Autodesk Inventor part; units mm, degrees
ref_plane "工作平面1" through (0, 165, 525) normal (0, 1, 0) x (1, 0, 0)
ref_plane "工作平面2" through (0, -340, 225) normal (0, 0, 1) x (1, 0, 0)
ref_plane "工作平面3" through (125, 0, 0) normal (1, 0, 0) x (0, 0, -1)
sketch "草图1" plane through (0, 0, 0) normal (1, 0, 0) x (0, 1, 0)
  line L0 (340, -525) -> (-340, -525)
  line L1 (-340, -525) -> (-340, 525)
  line L2 (-340, 525) -> (340, 525)
  line L3 (340, 525) -> (340, -525)
  line L4 (340, -525) -> (-340, 525) construction
  line L5 (-340, -525) -> (340, 525) construction
  point P0 (0, 0)
  dimension "d0" = 680
  dimension "d1" = 1050
extrude "拉伸1" add sketch "草图1" along normal blind 190
fillet "圆角1" [suppressed]
sketch "草图2" plane through (190, 0, 0) normal (1, 0, 0) x (0, 0, -1)
  line L0 (475, -290) -> (-475, -290)
  line L1 (475, 290) -> (475, -290)
  line L2 (-475, 290) -> (475, 290)
  line L3 (-475, -290) -> (-475, 290)
  line L4 (-475, 290) -> (475, 290)
  line L5 (475, 290) -> (475, 190)
  line L6 (475, 190) -> (-475, 190)
  line L7 (-475, 190) -> (-475, 290)
  point P0 (0, 0)
  dimension "d5" = 100
extrude "拉伸2" [suppressed]
sketch "草图3" plane through (190, 0, 0) normal (1, 0, 0) x (0, 0, -1)
  line L0 (-475, -290) -> (-475, 290)
  line L1 (475, -290) -> (-475, -290)
  line L2 (475, 290) -> (475, -290)
  line L3 (-525, -340) -> (525, -340)
  line L4 (-525, 340) -> (-525, -340)
  line L5 (525, -340) -> (525, 340)
  line L6 (-475, -241.0052) -> (375, -241.0052)
  line L7 (375, -241.0052) -> (375, -341.0052)
  line L8 (375, -341.0052) -> (-475, -341.0052)
  line L9 (-475, -341.0052) -> (-475, -241.0052)
  point P0 (0, 0)
  point P1 (425, -191.0052)
  point P2 (425, -240)
  dimension "d8" = 850
  dimension "d9" = 100
extrude "拉伸3" [suppressed]
sketch "草图4" plane through (190, -191.0052, -425) normal (0, -1, 0) x (1, 0, 0)
  line L0 (-27.3454, 1.363) -> (-107.3454, 1.363)
  line L1 (-107.3454, 1.363) -> (-107.3454, 851.363)
  line L2 (-107.3454, 851.363) -> (-27.3454, 851.363)
  line L3 (-27.3454, 851.363) -> (-27.3454, 1.363)
  point P0 (-190, 425)
  dimension "d12" = 80
  dimension "d13" = 850
extrude "拉伸4" [suppressed]
sketch "草图5" plane through (190, 0, 0) normal (1, 0, 0) x (0, 0, -1)
  line L0 (475, -290) -> (-475, -290)
  line L1 (475, 290) -> (475, -290)
  line L2 (-475, 290) -> (475, 290)
  line L3 (-475, -290) -> (-475, 290)
  line L4 (-400, -285) -> (400, -285)
  line L5 (400, -285) -> (400, -325)
  line L6 (400, -325) -> (-400, -325)
  line L7 (-400, -325) -> (-400, -285)
  line L8 (-525, -340) -> (525, -340)
  point P0 (0, 0)
  point P1 (-400, -305)
  point P2 (-400, -290)
  point P3 (400, -290)
  dimension "d16" = 800
  dimension "d17" = 40
  dimension "d19" = 75
  dimension "d34" = 55
extrude "拉伸5" cut sketch "草图5" against normal blind 105 contours L5 L6 L7 L0 | L0 L7 L4 L5
ref_plane "工作平面1" through (0, 165, 525) normal (0, 1, 0) x (1, 0, 0)
sketch "草图6" plane through (0, 165, 525) normal (0, 1, 0) x (1, 0, 0)
  line L0 (190, 50) -> (190, 1000)
  arc A0 (190, 1000) -> (140, 1050) centre (140, 1000) ccw
  line L1 (140, 1050) -> (140, 0)
  arc A1 (140, 0) -> (190, 50) centre (140, 50) ccw
  line L2 (0, 1050) -> (190, 1050)
  line L3 (0, 1050) -> (0, 0)
  line L4 (0, 0) -> (190, 0)
  line L5 (145, 150) -> (45, 150)
  line L6 (45, 150) -> (45, 900)
  line L7 (45, 900) -> (145, 900)
  line L8 (145, 900) -> (145, 150)
  line L9 (190, 1050) -> (190, 0)
  point P0 (0, 525)
  dimension "d23" = 100
  dimension "d24" = 750
  dimension "d25" = 150
  dimension "d26" = 45
extrude "拉伸6" cut sketch "草图6" against normal blind 450 contours L5 L6 L7 L1 | L1 L7 L8 L5
fillet "圆角3" [suppressed]
ref_plane "工作平面2" through (0, -340, 225) normal (0, 0, 1) x (1, 0, 0)
sketch "草图7" plane through (0, -340, 225) normal (0, 0, 1) x (1, 0, 0)
  point P0 (0, 340)
sketch "草图8" plane through (0, -340, 225) normal (0, 0, 1) x (1, 0, 0)
  line L0 (-8.4267, 713.5838) -> (252.801, 713.5838)
  line L1 (252.801, 713.5838) -> (252.801, -46.692)
  line L2 (252.801, -46.692) -> (-8.4267, -46.692)
  line L3 (-8.4267, -46.692) -> (-8.4267, 713.5838)
  point P0 (0, 340)
extrude "拉伸7" [suppressed]
sketch "草图9" plane through (190, -285, -400) normal (0, -1, 0) x (1, 0, 0)
  line L0 (0, 800) -> (-105, 800)
  line L1 (0, 0) -> (-105, 0)
  line L2 (-105, 0) -> (-105, 800)
  arc A0 (0, 875) -> (-50, 925) centre (-50, 875) ccw
  line L3 (0, 875) -> (-190, 875)
  line L4 (-190, -125) -> (-190, 925)
  arc A1 (-50, -125) -> (0, -75) centre (-50, -75) ccw
  line L5 (0, -75) -> (-190, -75)
  line L6 (-95, 875) -> (-95, -75)
  line L7 (-25, 800) -> (-65, 800)
  line L8 (-65, 800) -> (-65, 0)
  line L9 (-65, 0) -> (-25, 0)
  line L10 (-25, 0) -> (-25, 800)
  line L11 (-185, 800) -> (-145, 800)
  line L12 (-145, 800) -> (-145, 0)
  line L13 (-145, 0) -> (-185, 0)
  line L14 (-185, 0) -> (-185, 800)
  point P0 (-190, 400)
  point P1 (-14.2929, 800)
  point P2 (-14.2929, 0)
  point P3 (-25, 0)
  point P4 (-65, 800)
  dimension "d35" = 40
  dimension "d36" = 30
extrude "拉伸8" [suppressed]
ref_plane "工作平面3" through (125, 0, 0) normal (1, 0, 0) x (0, 0, -1)
sketch "草图10" plane through (125, 0, 0) normal (1, 0, 0) x (0, 0, -1)
  line L0 (400, -280) -> (-400, -280)
  line L1 (-400, -280) -> (-400, 220)
  line L2 (-400, 220) -> (400, 220)
  line L3 (400, -280) -> (400, 220)
  line L4 (-400, 220) -> (400, 220)
  line L5 (400, 220) -> (400, 160)
  line L6 (400, 160) -> (-400, 160)
  line L7 (-400, 160) -> (-400, 220)
  point P0 (0, 0)
  point P1 (-400, 160)
  point P2 (400, 160)
  dimension "d40" = 800
  dimension "d41" = 60
extrude "拉伸9" [suppressed]
fillet "圆角4" [suppressed]
ref_plane "工作平面4" through (190, -290, -400) normal (0, -1, 0) x (1, 0, 0)
ref_plane "工作平面5" through (95, 0, 0) normal (1, 0, 0) x (0, 0, -1)
ref_plane "工作平面6" through (190, -290, 350) normal (0, 0, -1) x (-1, 0, 0)
sketch "草图11" plane through (0, -340, -525) normal (0, 0, -1) x (-1, 0, 0)
  point P0 (0, 340)
ref_plane "工作平面7" through (0, -340, 225) normal (0, 0, 1) x (1, 0, 0)
sketch "草图12" plane through (0, -340, 225) normal (0, 0, 1) x (1, 0, 0)
  line L0 (145, 505) -> (45, 505)
  line L1 (145, 55) -> (85, 55)
  line L2 (145, 505) -> (145, 55)
  line L3 (145, 505) -> (45, 505)
  line L4 (45, 505) -> (45, 55)
  line L5 (45, 55) -> (85, 55)
  line L6 (190, 55) -> (190, 15)
  line L7 (190, 55) -> (85, 55)
  line L8 (85, 55) -> (85, 15)
  line L9 (190, 15) -> (85, 15)
  line L10 (0, 0) -> (190, 0)
  line L11 (0, 0) -> (0, 680)
  line L12 (0, 680) -> (190, 680)
  line L13 (190, 0) -> (190, 680)
  point P0 (0, 340)
sketch "草图13" plane through (0, -340, -525) normal (0, 0, -1) x (-1, 0, 0)
  line L0 (-45, 505) -> (-45, 55)
  line L1 (-45, 55) -> (-85, 55)
  line L2 (-85, 55) -> (-85, 15)
  line L3 (-85, 55) -> (-65, 55)
  line L4 (-65, 55) -> (-65, 15)
  line L5 (-65, 15) -> (-85, 15)
  line L6 (-85, 15) -> (-85, 55)
  point P0 (0, 340)
  point P1 (-65, 35)
  dimension "d49" = 20
  dimension "d50" = 40
  dimension "d51" = 20
extrude "拉伸10" [suppressed]
sketch "草图14" plane through (190, -325, 400) normal (0, 0, -1) x (-1, 0, 0)
  line L0 (145, 490) -> (45, 490)
  line L1 (45, 490) -> (45, 40)
  line L2 (105, 40) -> (45, 40)
  line L3 (105, 40) -> (145, 40)
  line L4 (145, 490) -> (145, 40)
  line L5 (0, 40) -> (0, 0)
  line L6 (0, 40) -> (105, 40)
  line L7 (105, 40) -> (105, 0)
  line L8 (0, 0) -> (105, 0)
  line L9 (105, 40) -> (85, 40)
  line L10 (85, 40) -> (85, 0)
  line L11 (85, 0) -> (105, 0)
  line L12 (105, 0) -> (105, 40)
  line L13 (45, 40) -> (65, 40)
  line L14 (65, 40) -> (65, 20)
  line L15 (65, 20) -> (45, 20)
  line L16 (45, 20) -> (45, 40)
  line L17 (145, 40) -> (105, 40)
  line L18 (105, 40) -> (125, 40)
  line L19 (125, 40) -> (125, 35)
  line L20 (125, 35) -> (105, 35)
  line L21 (105, 35) -> (105, 40)
  point P0 (190, 325)
  point P1 (85, 40)
  dimension "d54" = 20
  dimension "d55" = 40
  dimension "d56" = 20
  dimension "d57" = 20
  dimension "d67" = 20
  dimension "d68" = 5
extrude "拉伸11" add sketch "草图14" along normal blind 800 contours L2 L14 L15 L16 | L7 L8 L10 L2
sketch "草图15" plane through (190, -325, 400) normal (0, 0, -1) x (-1, 0, 0)
  line L0 (0, 40) -> (45, 40)
  line L1 (45, 40) -> (0, 40)
  line L2 (0, 40) -> (0, 35)
  line L3 (0, 35) -> (45, 35)
  line L4 (45, 35) -> (45, 40)
  point P0 (190, 325)
  dimension "d60" = 45
  dimension "d61" = 5
extrude "拉伸12" [suppressed]
sketch "草图16" plane through (190, -325, 400) normal (0, 1, 0) x (1, 0, 0)
  line L0 (-105, 800) -> (-105, 0)
  line L1 (0, 800) -> (0, 0)
  line L2 (-105, 0) -> (0, 0)
  line L3 (0, 0) -> (0, 800)
  line L4 (0, 800) -> (-105, 800)
  line L5 (-105, 800) -> (-105, 0)
  point P0 (-190, 400)
extrude "拉伸13" [suppressed]
fillet "圆角5" [suppressed]
sketch "草图17" plane through (190, -325, 400) normal (0, 0, -1) x (-1, 0, 0)
  line L0 (145, 40) -> (85, 40)
  line L1 (125, 40) -> (105, 40)
  line L2 (105, 40) -> (105, 35)
  line L3 (105, 35) -> (125, 35)
  line L4 (125, 35) -> (125, 40)
  line L5 (145, 490) -> (145, 40)
  point P0 (190, 325)
  point P1 (125, 37.5)
  point P2 (105, 40)
  dimension "d69" = 20
  dimension "d70" = 5
  dimension "d71" = 20
extrude "拉伸14" cut sketch "草图17" along normal blind 800
ref_plane "工作平面8" through (0, -340, 225) normal (0, 0, 1) x (1, 0, 0)
sketch "草图18" plane through (0, -340, 225) normal (0, 0, 1) x (1, 0, 0)
  line L0 (-8.4988, 711.8216) -> (199.7213, 711.8216)
  line L1 (199.7213, 711.8216) -> (199.7213, -36.0709)
  line L2 (199.7213, -36.0709) -> (-8.4988, -36.0709)
  line L3 (-8.4988, -36.0709) -> (-8.4988, 711.8216)
  point P0 (0, 340)
extrude "拉伸15" [suppressed]
sketch "草图19" plane through (145, -305, 400) normal (1, 0, 0) x (0, 0, -1)
  line L0 (0, 20) -> (25, 20)
  line L1 (0, 0) -> (800, 0)
  line L2 (0, 20) -> (800, 20)
  line L3 (800, 20) -> (800, 0)
  line L4 (800, 0) -> (0, 0)
  line L5 (0, 0) -> (0, 20)
  point P0 (400, 305)
extrude "拉伸16" [suppressed]
sketch "草图20" plane through (190, -325, 400) normal (0, 0, -1) x (-1, 0, 0)
  line L0 (65, 40) -> (85, 40)
  line L1 (65, 20) -> (45, 20)
  line L2 (65, 40) -> (45, 40)
  line L3 (45, 40) -> (45, 20)
  line L4 (45, 20) -> (65, 20)
  line L5 (65, 20) -> (65, 40)
  point P0 (190, 325)
extrude "拉伸17" cut sketch "草图20" along normal blind 800
properties part number "heater" material "聚碳酸酯，透明"
CAD build for the part. Positions are in the model's coordinates, mm. A direction names the side the tool comes from. Give positions to 0.01 mm unless a question says otherwise; leave off trailing zeros. Write each loop counter-clockwise with the first axis right and the second up, starting at its lowest first coordinate (ties: lowest second). Pieces come first, ordered by that corner, then holes. Notation, with made-up numbers: M 12.25,-21 L 46.25,-21 A19 cw 46.25,-12 Z; hole C 0,79 d3. An arc over 180 degrees is marked long. Put each result on its own line as item: value. Start each with the question number.
(1) Probe L1, parallel to Z at x = 57, y = -254; L2, parallel to X at y = -58, z = 20; L3, parallel to Y at x = 89.5, z = 153. List the from-to ranges inside material, lowest first.
(2) Band-saw the part on A-A, the plane y = 129.5. Write the cut outline in (x, z).
(3) Flat gauge pin, fed straight in: pin 1 Ø4 at (y, z) = (-288.5, -51) entering from +X. Where does the tip first touch, or does it go through?
(4) Band-saw the part on B-B, the plane x = 161. Write the cut outline in (y, z), and give its area (3 significant figures).
(5) Band-saw the part on C-C, the plane z = -125.5. Write the cut outline in (x, y).
(6) Mould opens along Y. For faces 4 (the face through (94, -340, -7)), 5 (the face through (190, -5, 7)), 6 (the face through (94, 340, 7)), 7 (the face through (45, -57, 5)) say: +Y half, -Y half, draft (parallel to the pull), parting line (faces both ways), or undercut.
(7) Which spindle directions (+Z, -Z, +X, -X, +Y, -Y) get a long thin tool onto all of the face, cutting with end or side? Do faces 1 (the face through (94, -57, -375)), 2 (the face through (94, -5, 525)), 3 (the face through (148, -305, 400)). Say none if no direction does.
Response values:
1. L1: z = -525 to -375, 375 to 525
1. L2: x = 0 to 45, 145 to 190
1. L3: y = -340 to -285, 165 to 340
2. outline: M 0,-525 L 190,-525 L 190,525 L 0,525 Z; hole M 45,-375 L 145,-375 L 145,375 L 45,375 Z
3. pin 1: stops at x = 105
4. outline: M -340,-525 L 340,-525 L 340,525 L -340,525 Z; hole M -325,-400 L -285,-400 L -285,400 L -325,400 Z
4. area: 682,000 mm2
5. outline: M 0,-340 L 190,-340 L 190,-325 L 105,-325 L 105,-285 L 85,-285 L 85,-290 L 65,-290 L 65,-285 L 45,-285 L 45,165 L 145,165 L 145,-285 L 190,-285 L 190,340 L 0,340 Z
6. face 4: -Y half
6. face 5: draft
6. face 6: +Y half
6. face 7: undercut
7. face 1: none
7. face 2: +Z, +X, -X, +Y, -Y
7. face 3: +X
